Part print with two shaded views. Sizes in mm from the minimum x, y, z corner. Give positions to 0.01 mm unless a question says otherwise; leave off trailing zeros. Write each loop counter-clockwise with the first axis right and the second up, starting at its lowest first coordinate (ties: lowest second). Pieces come first, ordered by that corner, then holes. Notation, with made-up numbers: (89.25, 39) - (134.25, 39) arc R12 cw to (134.25, 51) - close; hole circle Ø7 at (34, 81). An arc over 180 degrees is marked (long way). Answer as a JSON object with one key per item and string values. Group by question number.
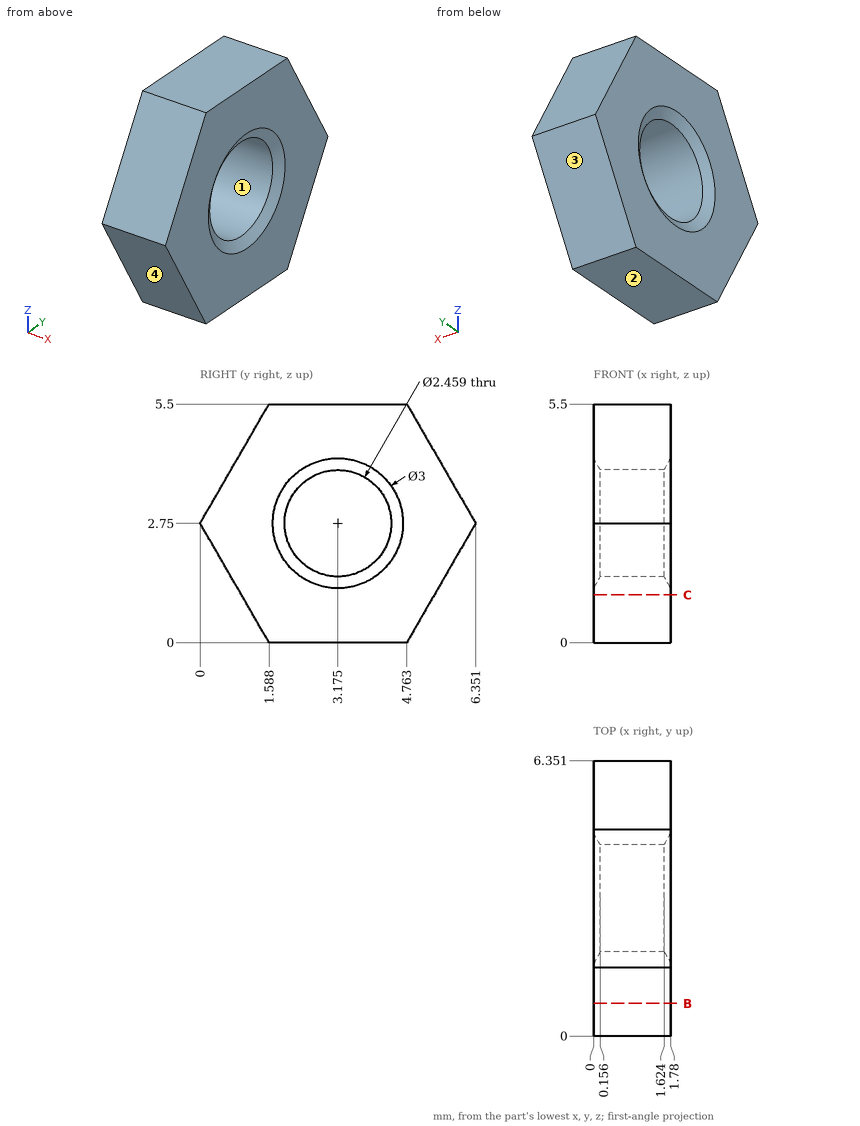
1) Saw through at B-B (y = 0.75). List the corners of the cut face in (x, z).
2) Drill centre lines: line 1 along Z through (x, y) = (1.15, 2.5); line 2 along Z through (x, y) = (0.6, 4); line 3 along Y through (x, z) = (1.4, 3.45) (1 decimal). Where is each one in solid material? Low to high. Write a range as from..to.
3) Two-plate mould, pull along Y, no slides. Class the marked faces 1, 2, 3 and 4: +Y half, -Y half, draft (parallel to the pull), parting line (faces both ways), or undercut.
4) Saw through at C-C (z = 1.1). List the corners of the cut face in (x, y).
Checks:
{
 "1": {"outline": "(0, 1.45) - (1.78, 1.45) - (1.78, 4.05) - (0, 4.05) - close"},
 "2": {"line 1": "0..1.72, 3.78..5.5", "line 2": "0..1.84, 3.66..5.5", "line 3": "0.4..2.2, 4.2..5.9"},
 "3": {"face 1": "undercut", "face 2": "draft", "face 3": "+Y half", "face 4": "-Y half"},
 "4": {"outline": "(0, 0.95) - (1.78, 0.95) - (1.78, 5.4) - (0, 5.4) - close"}
}
